Part model, mm, in its own coordinate system. A direction names the side the tool comes from. Give positions to 0.01 mm unless a question says otherwise; leave off trailing zeros. Loops run counter-clockwise (first coordinate to the right, second up) from the corner with the lowest first, then second, coordinate; pieces in that order, holes last. Notation, with made-up numbers: M 58.25,25.5 L 71.25,25.5 A22 ccw 71.25,58.5 Z; hole C -30,6.5 d7. An arc over 180 degrees is marked long. Put each result on its own line as item: value. Start each with the question number.
```python
from build123d import *

# Parameters (mm, degrees)
SKETCH1_W               = 30
SKETCH1_H               = 30
BOSS_EXTRUDE1_DEPTH     = 0.375
SKETCH2_R               = 1.3
CUT_EXTRUDE1_DEPTH      = 1.75
MIRROR2_COPY_1_SKETCH_R = 1.3
MIRROR2_COPY_1_DEPTH    = 1.75
SKETCH3_W               = 7.2
SKETCH3_H               = 9
SKETCH3_W_2             = 6
SKETCH3_H_2             = 8
BOSS_EXTRUDE2_DEPTH     = 3.2
FILLET1_R               = 2
FILLET2_R               = 0.5
SKETCH4_W               = 8
SKETCH4_H               = 1
BOSS_EXTRUDE3_DEPTH     = 0.5


with BuildPart() as part:
    # Sketch1 → Boss-Extrude1 (new body, symmetric)
    with BuildSketch(Plane(origin=(0, 0, 0), x_dir=(1, 0, 0), z_dir=(0, 1, 0))):
        Rectangle(SKETCH1_W, SKETCH1_H)
    extrude(amount=BOSS_EXTRUDE1_DEPTH, both=True)

    # Sketch2 → Cut-Extrude1 (cut, through all)
    with BuildSketch(Plane(origin=(0, 0.375, 0), x_dir=(1, 0, 0), z_dir=(0, 1, 0))):
        with Locations((-12.7, 12.7)):
            Circle(SKETCH2_R)
    cut_extrude1 = extrude(amount=-CUT_EXTRUDE1_DEPTH, mode=Mode.SUBTRACT)

    # Mirror1: Cut-Extrude1 across plane
    add(cut_extrude1.mirror(Plane(origin=(0, 0, 0), x_dir=(0, 0, 1), z_dir=(1, 0, 0))), mode=Mode.SUBTRACT)

    # Mirror2: Cut-Extrude1 across plane
    add(cut_extrude1.mirror(Plane.XY), mode=Mode.SUBTRACT)

    # Mirror2 copy 1 sketch → Mirror2 copy 1 (cut, through all)
    with BuildSketch(Plane(origin=(0, 0.375, 0), x_dir=(-1, 0, 0), z_dir=(0, 1, 0))):
        with Locations((-12.7, 12.7)):
            Circle(MIRROR2_COPY_1_SKETCH_R)
    extrude(amount=-MIRROR2_COPY_1_DEPTH, mode=Mode.SUBTRACT)

    # Sketch3 → Boss-Extrude2 (add)
    with BuildSketch(Plane(origin=(0, 0.375, 0), x_dir=(1, 0, 0), z_dir=(0, 1, 0))):
        with Locations((-11.4, -4.9)):
            Rectangle(SKETCH3_W, SKETCH3_H)
        with Locations((-12, 5.6)):
            Rectangle(SKETCH3_W_2, SKETCH3_H_2)
    extrude(amount=BOSS_EXTRUDE2_DEPTH)

    # Fillet1
    fillet1_edges = [part.edges().sort_by_distance(p)[0] for p in [
        (-11.4, 3.575, 9.4),
        (-11.4, 3.575, 0.4),
    ]]
    fillet(fillet1_edges, radius=FILLET1_R)

    # Fillet2
    fillet2_edges = [part.edges().sort_by_distance(p)[0] for p in [
        (-12, 3.575, -1.6),
        (-12, 3.575, -9.6),
    ]]
    fillet(fillet2_edges, radius=FILLET2_R)

    # Sketch4 → Boss-Extrude3 (add, symmetric)
    with BuildSketch(Plane(origin=(0, 0.375, 0), x_dir=(1, 0, 0), z_dir=(0, 1, 0))):
        with Locations((-6, 14.5)):
            Rectangle(SKETCH4_W, SKETCH4_H)
    extrude(amount=BOSS_EXTRUDE3_DEPTH, both=True)


solid = part.part
```
1) Pin check, flat tips, straight feed: pin 1 Ø4 at (x, z) = (-12.7, 12.7) entering from +Y (3 decimals); pin 2 Ø1.4 at (x, y) = (-13, 2.5) entering from -Z; pin 3 Ø1.6 at (y, z) = (1.5, -4.5) entering from +X. Stop position of each tip, or through.
2) Band-saw the part on C-C on z = 6.75. Give the cut face in (x, y) (3 decimals), then the cut area to 3 significant figures.
3) Mould opens along Z. For faces 5 (the flat face through (0, 0, -15)), 6 (the cylindrical face through (11.5, 0, 12.2)), 7 (the flat face through (-11, 3.575, 5)) say: +Z half, -Z half, draft (parallel to the pull), parting line (faces both ways), or undercut.
4) Which spindle directions (+Z, -Z, +X, -X, +Y, -Y) get a long thin tool onto all of the face, cutting with end or side? Do faces 1 (the flat face through (-6.1, 0.875, -14.5)), 2 (the flat face through (-15, 0, 0)), 3 (the flat face through (-11, 1, 9.4)), 4 (the flat face through (-12, 2, -1.6)). Say none if no direction does.
5) Band-saw the part on A-A on z = 12.7. Give the cut face in (x, y) (3 decimals), then the cut area to 3 significant figures.
6) Band-saw the part on D-D on x = -5.5. Give the cut face in (y, z) (3 decimals), then the cut area to 3 significant figures.
7) Wall check: L1, parallel to X at y = -0.15, z = -12.7; L2, parallel to Y at x = -4, z = 3.25 (3 decimals). Give the ranges that are in metal, low to high.
8) Band-saw the part on B-B on x = 12.7. Give the cut face in (y, z) (3 decimals), then the cut area to 3 significant figures.
Evaluation:
1. pin 1: y = 0.375
1. pin 2: z = -9.6
1. pin 3: x = -9
2. outline: M -15,-0.375 L 15,-0.375 L 15,0.375 L -7.8,0.375 L -7.8,3.575 L -15,3.575 Z
2. area: 45.5 mm2
3. face 5: -Z half
3. face 6: undercut
3. face 7: draft
4. face 1: -Z, +X, -X, +Y
4. face 2: +Z, -Z, -X, +Y, -Y
4. face 3: +Z, +X, -X, +Y
4. face 4: +X, -X, +Y
5. outline: M -15,-0.375 L -14,-0.375 L -14,0.375 L -15,0.375 Z; M -11.4,-0.375 L 11.4,-0.375 L 11.4,0.375 L -11.4,0.375 Z; M 14,-0.375 L 15,-0.375 L 15,0.375 L 14,0.375 Z
5. area: 18.6 mm2
6. outline: M -0.375,-15 L 0.875,-15 L 0.875,-14 L 0.375,-14 L 0.375,15 L -0.375,15 Z
6. area: 23.0 mm2
7. L1: -15 to -14, -11.4 to 11.4, 14 to 15
7. L2: -0.375 to 0.375
8. outline: M -0.375,-15 L 0.375,-15 L 0.375,-14 L -0.375,-14 Z; M -0.375,-11.4 L 0.375,-11.4 L 0.375,11.4 L -0.375,11.4 Z; M -0.375,14 L 0.375,14 L 0.375,15 L -0.375,15 Z
8. area: 18.6 mm2
